from build123d import *

# Parameters (mm, degrees)
BOSS_EXTRUDE2_DEPTH = 3.175


with BuildPart() as part:
    # Sketch1 → Boss-Extrude2 (new body)
    with BuildSketch(Plane.XY):
        Polygon((3.175, 20.6375), (3.175, 17.6276), (6.35, 17.6276), (6.35, 20.240625), (9.525, 20.240625), (9.525, 17.6276), (10.795, 17.6276), (10.795, 14.1224), (9.525, 14.1224), (9.525, 11.509375), (6.35, 11.509375), (6.35, 14.1224), (3.175, 14.1224), (3.175, 11.1125), (0, 11.1125), (0, 0), (12.3825, 0), (12.779375, 14.2875), (13.17625, 0), (13.9065, 0), (14.303375, 14.2875), (14.70025, 0), (15.4305, 0), (15.827375, 14.2875), (16.22425, 0), (16.9545, 0), (17.351375, 14.2875), (17.74825, 0), (18.4785, 0), (18.875375, 14.2875), (19.27225, 0), (20.0025, 0), (20.399375, 14.2875), (20.79625, 0), (21.5265, 0), (21.923375, 14.2875), (22.32025, 0), (23.0505, 0), (23.447375, 14.2875), (23.84425, 0), (24.5745, 0), (24.971375, 14.2875), (25.36825, 0), (26.0985, 0), (26.495375, 14.2875), (26.89225, 0), (27.6225, 0), (28.019375, 14.2875), (28.41625, 0), (29.1465, 0), (29.543375, 14.2875), (29.94025, 0), (30.6705, 0), (31.067375, 14.2875), (31.46425, 0), (32.1945, 0), (32.591375, 14.2875), (32.98825, 0), (33.7185, 0), (34.115375, 14.2875), (34.51225, 0), (34.925, 0), (34.925, -3.175), (36.5125, -3.175), (36.5125, 0), (38.1, 0), (38.1, 31.75), (36.5125, 31.75), (36.5125, 34.925), (34.925, 34.925), (34.925, 31.75), (34.51225, 31.75), (34.115375, 17.4625), (33.7185, 31.75), (32.98825, 31.75), (32.591375, 17.4625), (32.1945, 31.75), (31.46425, 31.75), (31.067375, 17.4625), (30.6705, 31.75), (29.94025, 31.75), (29.543375, 17.4625), (29.1465, 31.75), (28.41625, 31.75), (28.019375, 17.4625), (27.6225, 31.75), (26.89225, 31.75), (26.495375, 17.4625), (26.0985, 31.75), (25.36825, 31.75), (24.971375, 17.4625), (24.5745, 31.75), (23.84425, 31.75), (23.447375, 17.4625), (23.0505, 31.75), (22.32025, 31.75), (21.923375, 17.4625), (21.5265, 31.75), (20.79625, 31.75), (20.399375, 17.4625), (20.0025, 31.75), (19.27225, 31.75), (18.875375, 17.4625), (18.4785, 31.75), (17.74825, 31.75), (17.351375, 17.4625), (16.9545, 31.75), (16.22425, 31.75), (15.827375, 17.4625), (15.4305, 31.75), (14.70025, 31.75), (14.303375, 17.4625), (13.9065, 31.75), (13.17625, 31.75), (12.779375, 17.4625), (12.3825, 31.75), (0, 31.75), (0, 20.6375), align=None)
        Polygon((13.17625, 15.875), (13.573125, 30.1625), (13.97, 15.875), (13.573125, 1.5875), align=None, mode=Mode.SUBTRACT)
        Polygon((14.70025, 15.875), (15.097125, 30.1625), (15.494, 15.875), (15.097125, 1.5875), align=None, mode=Mode.SUBTRACT)
        Polygon((16.22425, 15.875), (16.621125, 30.1625), (17.018, 15.875), (16.621125, 1.5875), align=None, mode=Mode.SUBTRACT)
        Polygon((17.74825, 15.875), (18.145125, 30.1625), (18.542, 15.875), (18.145125, 1.5875), align=None, mode=Mode.SUBTRACT)
        Polygon((19.27225, 15.875), (19.669125, 30.1625), (20.066, 15.875), (19.669125, 1.5875), align=None, mode=Mode.SUBTRACT)
        Polygon((20.79625, 15.875), (21.193125, 30.1625), (21.59, 15.875), (21.193125, 1.5875), align=None, mode=Mode.SUBTRACT)
        Polygon((22.32025, 15.875), (22.717125, 30.1625), (23.114, 15.875), (22.717125, 1.5875), align=None, mode=Mode.SUBTRACT)
        Polygon((23.84425, 15.875), (24.241125, 30.1625), (24.638, 15.875), (24.241125, 1.5875), align=None, mode=Mode.SUBTRACT)
        Polygon((25.36825, 15.875), (25.765125, 30.1625), (26.162, 15.875), (25.765125, 1.5875), align=None, mode=Mode.SUBTRACT)
        Polygon((26.89225, 15.875), (27.289125, 30.1625), (27.686, 15.875), (27.289125, 1.5875), align=None, mode=Mode.SUBTRACT)
        Polygon((28.41625, 15.875), (28.813125, 30.1625), (29.21, 15.875), (28.813125, 1.5875), align=None, mode=Mode.SUBTRACT)
        Polygon((29.94025, 15.875), (30.337125, 30.1625), (30.734, 15.875), (30.337125, 1.5875), align=None, mode=Mode.SUBTRACT)
        Polygon((31.46425, 15.875), (31.861125, 30.1625), (32.258, 15.875), (31.861125, 1.5875), align=None, mode=Mode.SUBTRACT)
        Polygon((32.98825, 15.875), (33.385125, 30.1625), (33.782, 15.875), (33.385125, 1.5875), align=None, mode=Mode.SUBTRACT)
        Polygon((34.51225, 15.875), (34.909125, 30.1625), (35.306, 15.875), (34.909125, 1.5875), align=None, mode=Mode.SUBTRACT)
    extrude(amount=BOSS_EXTRUDE2_DEPTH)


solid = part.part
Source: CAD feature listing. Evaluate the final solid. Frame: model axes, mm. Round coordinates to 2 decimals unless told otherwise and drop trailing zeros. One line per item, written item: value. Start each with the question number.
Item 1: Section query A-A (z = 2.55). State how many separate pieces and enclosed holes the cut face has, plus the area to 3 significant figures.
Item 2: Mould query, pull axis X, two halves, no side actions, for faces 1 (the flat face through (3.175, 19, 2)), 2 (the flat face through (9.525, 19, 2)). Classes: pulls with the +X half, pulls with the -X half, needs draft (parallel to the pull), parting line crosses it, or undercut.
Item 3: Ray query, L1, parallel to Y at x = 4.5, z = 2.65; L2, parallel to Y at x = 8, z = 0.9; L3, parallel to X at y = 33, z = 1.2 (1 decimal). Return the intervals inside material, ascending. Write a range as from..to.
Item 4: Pin query (flat end, axial travel): pin 1 (1.6 mm diameter, centred on y = -2, z = 1.5, fed in from +X); pin 2 (0.6 mm diameter, centred on x = 30.5, z = 1, fed in from -Y); pin 3 (1.5 mm diameter, centred on y = 12, z = 1.5, fed in from -X) (3 decimals). Return the tip coordinate at first contact, or that it passes through.
Result set:
1. separate pieces: 1
1. enclosed holes: 15
1. area: 806 mm²
2. face 1: pulls with the -X half
2. face 2: undercut
3. L1: y = 0..14.12, 17.63..31.75
3. L2: y = 0..11.51, 20.24..31.75
3. L3: x = 34.9..36.5
4. pin 1: stops at x = 36.51
4. pin 2: stops at y = 0
4. pin 3: stops at x = 3.175
